Read the model definition and answer for the solid it produces. Units are mm, in the model's axes. Face numbers are marked on the shaded views. A direction names the side the tool comes from. Round coordinates to 2 decimals unless told otherwise and drop trailing zeros. Order: outer loops, then holes, each group sorted by start corner. A loop starts at its lowest first (then second) coordinate and runs counter-clockwise, first axis right, second up. Notation, with made-up numbers: (89, -34.5) - (93, -34.5) arc R16 cw to (93, -28.5) - close; hole circle Ø7 at (74.5, -39.5). An arc over 180 degrees is marked (long way). One line per question, with ' | ' between items. Start each with the question number.
1) The part is cut by section D-D, the plane x = -60.5. Give the vertices of the cut face in (y, z), plus the area to 3 significant figures.
2) The part is cut by section A-A, the plane y = 3.25. Give the vertices of the cut face in (x, z), plus the area to 3 significant figures.
3) The part is cut by section B-B, the plane z = 21. Give the vertices of the cut face in (x, y), plus the area to 3 significant figures.
4) The mould has two halves that part along X. Classify the marked faces 4, 5 and 6: pulls with the +X half, pulls with the -X half, needs draft (parallel to the pull), parting line crosses it, or undercut.
5) Straight lines are drawn through the part: line 1 (X direction, y = 12.5, z = -12); line 2 (Z direction, x = 1, y = 16); line 3 (Y direction, x = -58, z = 16). For each, find the intervals that lie inside material, in ascending order. Write a range as from..to.
6) For the marked faces 1, 2 and 3, determine the directions among +Z, -Z, +X, -X, +Y, -Y from which every point of the face is accessible in a straight line to the end or side of a thin tool.
7) The part is cut by section C-C, the plane x = -5.5. Give the vertices of the cut face in (y, z).
8) Flat-ended cylindrical pins translate along their axes: pin 1 (5.5 mm diameter, centred on y = 3, z = 48, fed in from -X); pin 2 (11 mm diameter, centred on x = -12, y = 13, fed in from +Z); pin 3 (5 mm diameter, centred on x = -18, z = -3, fed in from +Y); pin 4 (4 mm diameter, centred on x = -52, z = 19, fed in from -Y). Find the tip coordinate at first contact, or state that the pin passes through.
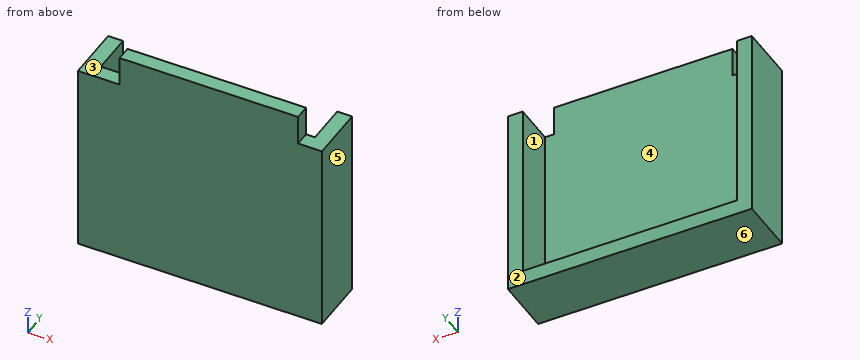
from build123d import *

# Parameters (mm, degrees)
EXTRUSION1_DEPTH = 5
EXTRUSION2_DEPTH = 14


with BuildPart() as part:
    # Esquisse1 → Extrusion1 (new body)
    with BuildSketch(Plane(origin=(0, 0, 0), x_dir=(1, 0, 0), z_dir=(0, 1, 0))):
        Polygon((-69.191486621, -43.16817348), (-55.191486621, -43.16817348), (-55.191486621, -53.16817348), (4.808513379, -53.16817348), (4.808513379, -43.16817348), (12.808513379, -43.16817348), (12.808513379, 21.83182652), (-69.191486621, 21.83182652), align=None)
    extrude(amount=EXTRUSION1_DEPTH)

    # Esquisse2 → Extrusion2 (add)
    with BuildSketch(Plane(origin=(0, 5, 0), x_dir=(1, 0, 0), z_dir=(0, 1, 0))):
        Polygon((12.808513379, -43.16817348), (12.808513379, 21.83182652), (-69.191486621, 21.83182652), (-69.191486621, -43.16817348), (-64.191486621, -43.16817348), (-64.191486621, 16.83182652), (7.808513379, 16.83182652), (7.808513379, -43.16817348), align=None)
    extrude(amount=EXTRUSION2_DEPTH)


solid = part.part
Values:
1) outline: (0, -21.83) - (19, -21.83) - (19, -16.83) - (5, -16.83) - (5, 43.17) - (0, 43.17) - close | area: 395 mm^2
2) outline: (-69.19, -21.83) - (12.81, -21.83) - (12.81, 43.17) - (4.81, 43.17) - (4.81, 53.17) - (-55.19, 53.17) - (-55.19, 43.17) - (-69.19, 43.17) - close | area: 5,930 mm^2
3) outline: (-69.19, 0) - (12.81, 0) - (12.81, 19) - (7.81, 19) - (7.81, 5) - (-64.19, 5) - (-64.19, 19) - (-69.19, 19) - close | area: 550 mm^2
4) face 4: undercut | face 5: pulls with the +X half | face 6: needs draft
5) line 1: x = -69.19..-64.19, 7.81..12.81 | line 2: z = -21.83..-16.83 | line 3: y = 0..5
6) face 1: +Z, +Y | face 2: +Z, -Z, +X, -X, +Y | face 3: +Z, -X, +Y, -Y
7) outline: (0, -21.83) - (19, -21.83) - (19, -16.83) - (5, -16.83) - (5, 53.17) - (0, 53.17) - close
8) pin 1: stops at x = -55.19 | pin 2: stops at z = -16.83 | pin 3: stops at y = 5 | pin 4: stops at y = 0
